Print and shaded views of the part. All mm, measured from the part's lowest x, y and z. A direction names the side the tool comes from. Coordinates: 2 decimals unless noted, no trailing zeros. Loops run counter-clockwise (first coordinate to the right, second up) from the corner with the lowest first, then second, coordinate; pieces in that order, holes last. Notation, with made-up numbers: M 55,21 L 59,21 A21 cw 59,49 Z; hole C 73.25,-39.5 d7. An arc over 180 degrees is marked long. Use a Markdown table: item, result. Add a question column.
1) Band-saw the part on D-D (y = 11.5). List the corners of the cut face in (x, z) (1 decimal).
2) Wall check: probe 1 along X at (y, z) = (3.25, 5.75) (1 decimal); probe 2 along Y at (x, z) = (1, 6.75); probe 3 along Y at (x, z) = (5.5, 4.5). Give the ranges that are in metal, low to high. Write a range as from..to.
3) Pin check, flat tips, straight feed: pin 1 Ø1 at (y, z) = (3.5, 4) entering from +X; pin 2 Ø1 at (y, z) = (3.5, 4) entering from -X (1 decimal); pin 3 Ø3 at (x, y) = (7.5, 13) entering from -Z. Stop position of each tip, or through.
4) Band-saw the part on B-B (z = 7.5). List the corners of the cut face in (x, y) (1 decimal).
5) Pull direction X, two halves, no side cores. Call the marked faces 4, 5 and 6: released by +X, released by -X, zero draft, split by the parting line, or undercut.
6) Tool access for the marked faces 1, 2 and 3: list every direction of +Z, -Z, +X, -X, +Y, -Y with a clear straight run to the whole face (end or side of a thin tool).
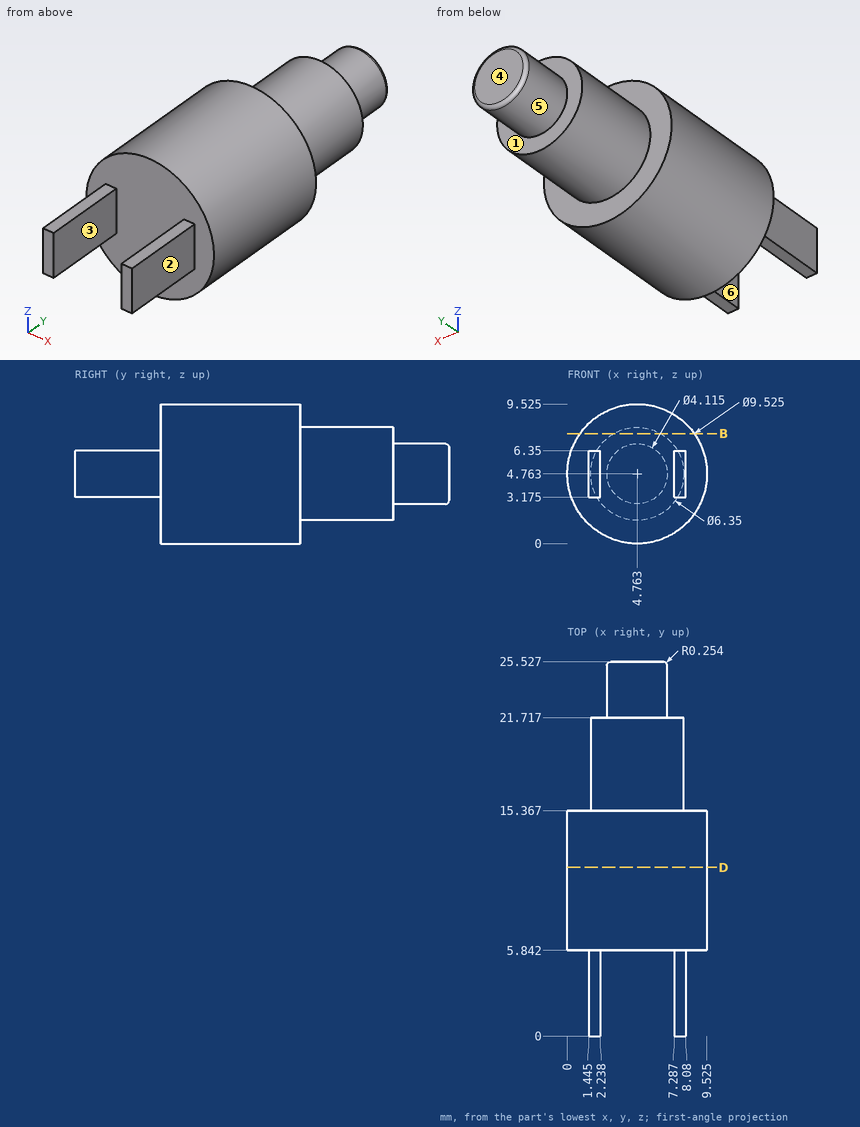
Entries:
| question | item | result |
|---|---|---|
| 1 | outline | C 4.8,4.8 d9.5 |
| 2 | probe 1 | 1.4..2.2, 7.3..8.1 |
| 2 | probe 2 | 5.84..15.37 |
| 2 | probe 3 | 5.84..25.53 |
| 3 | pin 1 | x = 8.08 |
| 3 | pin 2 | x = 1.4 |
| 3 | pin 3 | z = 0.16 |
| 4 | outline | M 0.9,5.8 L 8.7,5.8 L 8.7,15.4 L 6.4,15.4 L 6.4,21.7 L 3.2,21.7 L 3.2,15.4 L 0.9,15.4 Z |
| 5 | face 4 | zero draft |
| 5 | face 5 | split by the parting line |
| 5 | face 6 | undercut |
| 6 | face 1 | +Y |
| 6 | face 2 | +Z, -Z, +X, -Y |
| 6 | face 3 | +Z, -Z, -Y |
